Geometry check sheet. Reference: the model listing, model coordinates, mm. A direction names the side the tool comes from. Round coordinates to 2 decimals unless told otherwise and drop trailing zeros. Order: outer loops, then holes, each group sorted by start corner. A loop starts at its lowest first (then second) coordinate and runs counter-clockwise, first axis right, second up. Notation, with made-up numbers: M 41,-9.75 L 97,-9.75 A7 ccw 97,-4.75 Z; hole C 19.25,86 d4. An arc over 180 degrees is marked long. Return JSON: item names as keys, results as strings. Group by question number.
```python
from build123d import *

# Parameters (mm, degrees)
F0_W      = 50.8
F0_H      = 38.1
F1_DEPTH  = 6.35
F2_W      = 44.45
F2_H      = 38.1
F3_DEPTH  = 19.05
F4_W      = 6.35
F4_H      = 19.05
F6_W      = 30.563162
F6_H      = 19.685
F7_DEPTH  = 7.62
F8_W      = 15.748
F8_H      = 19.05
F9_DEPTH  = 7.112
F10_W     = 12.7
F10_H     = 19.05
F11_DEPTH = 7.112
F12_R     = 5.08
F13_R     = 5.08


with BuildPart() as f1:
    # F0 (on Top) → F1 (new body)
    with BuildSketch(Plane.XY):
        Rectangle(F0_W, F0_H)
    extrude(amount=F1_DEPTH)

    # F2 (on face) → F3 (join)
    with BuildSketch(Plane.XY.offset(6.35)):
        Rectangle(F2_W, F2_H)
    extrude(amount=F3_DEPTH)

    # F4 (on Right) → F5 (revolve, cut)
    with BuildSketch(Plane.YZ):
        with Locations((-18.92219, 16.263971)):
            Rectangle(F4_W, F4_H)
    revolve(axis=Axis((0, -15.74719, 16.263971), (0, 0, 1)), mode=Mode.SUBTRACT)

    # F6 (on face) → F7 (cut)
    with BuildSketch(Plane(origin=(0, 19.05, 0), x_dir=(-1, 0, 0), z_dir=(0, 1, 0))):
        with Locations((0, 15.5575)):
            Rectangle(F6_W, F6_H)
    extrude(amount=-F7_DEPTH, mode=Mode.SUBTRACT)

    # F8 (on face) → F9 (cut)
    with BuildSketch(Plane(origin=(-22.225, 0, 0), x_dir=(0, -1, 0), z_dir=(-1, 0, 0))):
        with Locations((11.176, 15.875)):
            Rectangle(F8_W, F8_H)
    extrude(amount=-F9_DEPTH, mode=Mode.SUBTRACT)

    # F10 (on face) → F11 (cut)
    with BuildSketch(Plane.YZ.offset(22.225)):
        with Locations((-12.7, 15.875)):
            Rectangle(F10_W, F10_H)
    extrude(amount=-F11_DEPTH, mode=Mode.SUBTRACT)

    # F12
    f12_edges = [f1.edges().sort_by_distance(p)[0] for p in [
        (-15.113, -3.302, 15.875),
    ]]
    fillet(f12_edges, radius=F12_R)

    # F13
    f13_edges = [f1.edges().sort_by_distance(p)[0] for p in [
        (15.113, -6.35, 15.875),
    ]]
    fillet(f13_edges, radius=F13_R)


solid = f1.part
```
Q1. Section check A-A on x = 0. Record the cut outline in (y, z) (3 decimals).
Q2. Material ranges on line 1 along X through (y, z) = (15, 19) (3 decimals); line 2 along Z through (x, y) = (-15, 17) (3 decimals); line 3 along Y through (x, z) = (0, 18), recorded low to high.
Q3. Section check D-D on x = -7.5. Record the cut outline in (y, z) (3 decimals).
Q4. Set-up check for faces 1 (the face through (0, 15, 5.715)), 2 (the face through (-22.225, 8, 16)), 3 (the face through (15.113, -15, 16)), 4 (the face through (-21, -3.302, 16)), 5 (the face through (0.2, -9.4, 16.2)): record each of +Z, -Z, +X, -X, +Y, -Y from which the full face is reachable in a straight line by a thin tool's end or side.
Q5. Depth check by flat-ended pin: pin 1 Ø8.5 at (y, z) = (-16, 19.5) entering from +X; pin 2 Ø5 at (y, z) = (-8.5, 11.5) entering from -X; pin 3 Ø5.5 at (y, z) = (-16.5, 20.5) entering from -X. Enter the tip coordinate at first touch or a pass-through.
Q6. Release check for a two-part mould opening along X. For faces 6 (the face through (0, 0, 0)), 7 (the face through (-25.4, 0, 3)), 8 (the face through (15.282, 15, 15)) record: +X half, -X half, draft (parallel to the pull), parting line (faces both ways), or undercut.
Q7. Section check C-C on z = 11. Record the cut outline in (x, y) (3 decimals), plus the area to 3 significant figures.
Q8. Section check B-B on y = 3. Record the cut outline in (x, z) (3 decimals).
Geometry check:
{
 "1": {"outline": "M -19.05,0 L 19.05,0 L 19.05,5.715 L 11.43,5.715 L 11.43,25.4 L -9.397,25.4 L -9.397,6.739 L -19.05,6.739 Z"},
 "2": {"line 1": "x = -22.225 to -15.282, 15.282 to 22.225", "line 2": "z = 0 to 5.715", "line 3": "y = -9.4 to 11.43"},
 "3": {"outline": "M -19.05,0 L 19.05,0 L 19.05,5.715 L 11.43,5.715 L 11.43,25.4 L -19.05,25.4 Z"},
 "4": {"face 1": "+Z, +Y", "face 2": "+Z, -X, +Y, -Y", "face 3": "+Z, +X, -Y", "face 4": "+Z, -X, -Y", "face 5": "+Z"},
 "5": {"pin 1": "stops at x = 15.11", "pin 2": "stops at x = -15.71", "pin 3": "stops at x = -15.11"},
 "6": {"face 6": "draft", "face 7": "-X half", "face 8": "undercut"},
 "7": {"outline": "M -22.225,-3.302 L -20.193,-3.302 A5.08 cw -15.113,-8.382 L -15.113,-19.05 L -5.423,-19.05 A6.35 cw long 5.423,-19.05 L 15.113,-19.05 L 15.113,-11.43 A5.08 cw 20.193,-6.35 L 22.225,-6.35 L 22.225,19.05 L 15.282,19.05 L 15.282,11.43 L -15.282,11.43 L -15.282,19.05 L -22.225,19.05 Z", "area": "1,170 mm^2"},
 "8": {"outline": "M -25.4,0 L 25.4,0 L 25.4,6.35 L 22.225,6.35 L 22.225,25.4 L -22.225,25.4 L -22.225,6.35 L -25.4,6.35 Z"}
}
